Check sheet for the drawn part. Datum: minimum x, y, z corner. Units: mm. Coordinates: 2 decimals unless noted, no trailing zeros. Order: outer loops, then holes, each group sorted by start corner. A loop starts at its lowest first (then second) coordinate and runs counter-clockwise, first axis right, second up.
Q1. Cross-section at A-A, the plane x = 3.25. Record the boundary of the cut face in (y, z), and give its area (3 significant figures).
Q2. Depth check by flat-ended pin: P1, Ø2, axis at x = 17.5, z = 30.5, coming from the -Y side; P2, Ø8, axis at x = 12.5, z = 26, coming from the -Y side. Enter the tip coordinate at first touch or a pass-through.
Q3. Cross-section at C-C, the plane x = 17. Record the boundary of the cut face in (y, z), and give its area (3 significant figures).
Q4. Thickness scan on line 1 (Z direction, x = 17.5, y = 1.4); line 2 (X direction, y = 0.2, z = 29.5); line 3 (Z direction, x = 18.25, y = 0.8). Record the ranges inside material, lowest first.
Q5. Cross-section at B-B, the plane y = 0.3. Record the boundary of the cut face in (x, z).
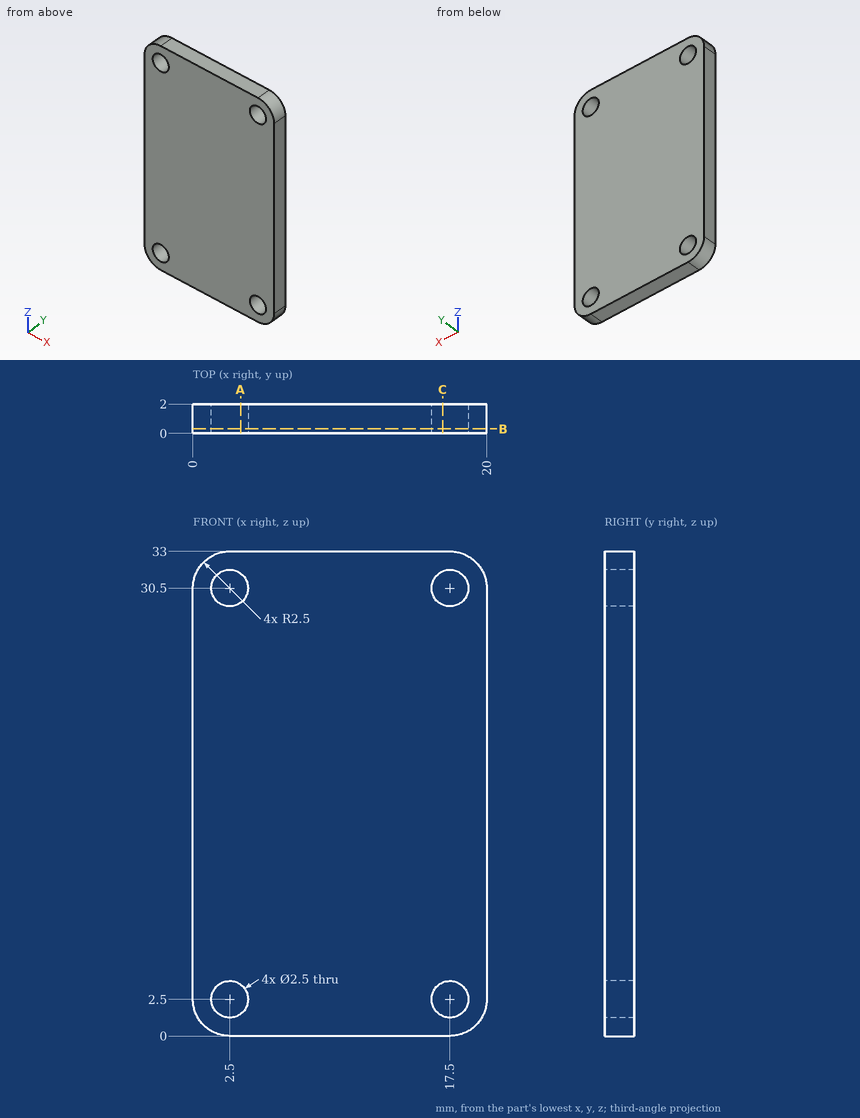
Check values:
1. outline: (0, 0) - (2, 0) - (2, 1.5) - (0, 1.5) - close; (0, 3.5) - (2, 3.5) - (2, 29.5) - (0, 29.5) - close; (0, 31.5) - (2, 31.5) - (2, 33) - (0, 33) - close
1. area: 58.0 mm2
2. P1: passes through
2. P2: stops at y = 0
3. outline: (0, 0) - (2, 0) - (2, 1.35) - (0, 1.35) - close; (0, 3.65) - (2, 3.65) - (2, 29.35) - (0, 29.35) - close; (0, 31.65) - (2, 31.65) - (2, 33) - (0, 33) - close
3. area: 56.8 mm2
4. line 1: z = 0 to 1.25, 3.75 to 29.25, 31.75 to 33
4. line 2: x = 0 to 1.75, 3.25 to 16.75, 18.25 to 20
4. line 3: z = 0.12 to 1.5, 3.5 to 29.5, 31.5 to 32.88
5. outline: (0, 2.5) arc R2.5 ccw to (2.5, 0) - (17.5, 0) arc R2.5 ccw to (20, 2.5) - (20, 30.5) arc R2.5 ccw to (17.5, 33) - (2.5, 33) arc R2.5 ccw to (0, 30.5) - close; hole circle Ø2.5 at (2.5, 2.5); hole circle Ø2.5 at (2.5, 30.5); hole circle Ø2.5 at (17.5, 2.5); hole circle Ø2.5 at (17.5, 30.5)
